from build123d import *

# Parameters (mm, degrees)
SKETCH1_W             = 425.069
SKETCH1_H             = 9.525
BOSS_EXTRUDE1_DEPTH   = 3.175
SKETCH2_W             = 3.175
SKETCH2_H             = 3.175
CUT_EXTRUDE1_DEPTH    = 213.611560649
SKETCH3_R             = 0.5
CUT_EXTRUDE2_DEPTH    = 213.611560649
SKETCH_PATTERN1_DEPTH = 3.175
SKETCH5_W             = 20
SKETCH5_H             = 3.18
BOSS_EXTRUDE2_DEPTH   = 3.175
SKETCH6_R             = 0.5
CUT_EXTRUDE3_DEPTH    = 213.706552841
SKETCH_PATTERN2_DEPTH = 3.175


# Read off the part's stored shape, not the designer's step: Sketch-Pattern1, Sketch-Pattern2
with BuildPart() as part:
    # Sketch1 → Boss-Extrude1 (new body)
    with BuildSketch(Plane(origin=(0, 0, 0), x_dir=(1, 0, 0), z_dir=(0, 1, 0))):
        Rectangle(SKETCH1_W, SKETCH1_H)
    extrude(amount=BOSS_EXTRUDE1_DEPTH)

    # Sketch2 → Cut-Extrude1 (cut, symmetric)
    with BuildSketch(Plane(origin=(0, 3.175, 0), x_dir=(1, 0, 0), z_dir=(0, 1, 0))):
        with Locations((-105.4735, 3.175)):
            Rectangle(SKETCH2_W, SKETCH2_H)
        with Locations((-210.947, 3.175)):
            Rectangle(SKETCH2_W, SKETCH2_H)
        with Locations((0, 3.175)):
            Rectangle(SKETCH2_W, SKETCH2_H)
    cut_extrude1 = extrude(amount=CUT_EXTRUDE1_DEPTH, both=True, mode=Mode.SUBTRACT)

    # Sketch3 → Cut-Extrude2 (cut, symmetric)
    with BuildSketch(Plane(origin=(0, 3.175, 0), x_dir=(1, 0, 0), z_dir=(0, 1, 0))):
        with Locations((-209.713053391, 1.941053391)):
            Circle(SKETCH3_R)
    cut_extrude2 = extrude(amount=CUT_EXTRUDE2_DEPTH, both=True, mode=Mode.SUBTRACT)

    # Mirror1: Cut-Extrude1 across plane
    add(cut_extrude1.mirror(Plane(origin=(0, 0, 0), x_dir=(0, 0, 1), z_dir=(1, 0, 0))), mode=Mode.SUBTRACT)

    # Sketch-Pattern1 outline → Sketch-Pattern1 (cut)
    with BuildSketch(Plane(origin=(0, 0, 0), x_dir=(1, 0, 0), z_dir=(0, 1, 0))):
        with BuildLine():
            Line((-103.886, 1.5875), (-104.593106781, 1.5875))
            ThreePointArc((-104.593106781, 1.5875), (-104.23955339, 1.441053391), (-103.886, 1.5875))
        make_face()
        with BuildLine():
            Line((-103.886, 2.294606781), (-103.886, 1.5875))
            ThreePointArc((-103.886, 1.5875), (-103.739553391, 1.941053391), (-103.886, 2.294606781))
        make_face()
        with BuildLine():
            Line((107.061, 1.5875), (106.353893219, 1.5875))
            ThreePointArc((106.353893219, 1.5875), (106.70744661, 1.441053391), (107.061, 1.5875))
        make_face()
        with BuildLine():
            Line((107.061, 2.294606781), (107.061, 1.5875))
            ThreePointArc((107.061, 1.5875), (107.207446609, 1.941053391), (107.061, 2.294606781))
        make_face()
        with BuildLine():
            Line((1.5875, 1.5875), (0.880393219, 1.5875))
            ThreePointArc((0.880393219, 1.5875), (1.23394661, 1.441053391), (1.5875, 1.5875))
        make_face()
        with BuildLine():
            Line((1.5875, 2.294606781), (1.5875, 1.5875))
            ThreePointArc((1.5875, 1.5875), (1.733946609, 1.941053391), (1.5875, 2.294606781))
        make_face()
    sketch_pattern1 = extrude(amount=SKETCH_PATTERN1_DEPTH, mode=Mode.SUBTRACT)

    # Mirror2: Cut-Extrude2, Sketch-Pattern1 across plane
    add(cut_extrude2.mirror(Plane(origin=(0, 0, 0), x_dir=(0, 0, 1), z_dir=(1, 0, 0))), mode=Mode.SUBTRACT)
    add(sketch_pattern1.mirror(Plane(origin=(0, 0, 0), x_dir=(0, 0, 1), z_dir=(1, 0, 0))), mode=Mode.SUBTRACT)

    # Sketch5 → Boss-Extrude2 (add)
    with BuildSketch(Plane(origin=(0, 3.175, 0), x_dir=(1, 0, 0), z_dir=(0, 1, 0))):
        with Locations((-158.21025, -6.3525)):
            Rectangle(SKETCH5_W, SKETCH5_H)
        with Locations((-52.73675, -6.3525)):
            Rectangle(SKETCH5_W, SKETCH5_H)
        with Locations((52.73675, -6.3525)):
            Rectangle(SKETCH5_W, SKETCH5_H)
        with Locations((158.21025, -6.3525)):
            Rectangle(SKETCH5_W, SKETCH5_H)
    extrude(amount=-BOSS_EXTRUDE2_DEPTH)

    # Sketch6 → Cut-Extrude3 (cut, symmetric)
    with BuildSketch(Plane(origin=(0, 3.175, 0), x_dir=(1, 0, 0), z_dir=(0, 1, 0))):
        with Locations((-168.563803391, -5.116053391)):
            Circle(SKETCH6_R)
    cut_extrude3 = extrude(amount=CUT_EXTRUDE3_DEPTH, both=True, mode=Mode.SUBTRACT)

    # Sketch-Pattern2 outline → Sketch-Pattern2 (cut)
    with BuildSketch(Plane(origin=(0, 0, 0), x_dir=(1, 0, 0), z_dir=(0, 1, 0))):
        with BuildLine():
            Line((-62.73675, -4.7625), (-62.73675, -5.469606781))
            ThreePointArc((-62.73675, -5.469606781), (-62.590303391, -5.116053391), (-62.73675, -4.7625))
        make_face()
        with BuildLine():
            Line((-63.443856781, -4.7625), (-62.73675, -4.7625))
            ThreePointArc((-62.73675, -4.7625), (-63.09030339, -4.616053391), (-63.443856781, -4.7625))
        make_face()
        with BuildLine():
            Line((148.21025, -4.7625), (148.21025, -5.469606781))
            ThreePointArc((148.21025, -5.469606781), (148.356696609, -5.116053391), (148.21025, -4.7625))
        make_face()
        with BuildLine():
            Line((147.503143219, -4.7625), (148.21025, -4.7625))
            ThreePointArc((148.21025, -4.7625), (147.85669661, -4.616053391), (147.503143219, -4.7625))
        make_face()
        with BuildLine():
            Line((42.73675, -4.7625), (42.73675, -5.469606781))
            ThreePointArc((42.73675, -5.469606781), (42.883196609, -5.116053391), (42.73675, -4.7625))
        make_face()
        with BuildLine():
            Line((42.029643219, -4.7625), (42.73675, -4.7625))
            ThreePointArc((42.73675, -4.7625), (42.38319661, -4.616053391), (42.029643219, -4.7625))
        make_face()
    sketch_pattern2 = extrude(amount=SKETCH_PATTERN2_DEPTH, mode=Mode.SUBTRACT)

    # Mirror3: Cut-Extrude3, Sketch-Pattern2 across plane
    add(cut_extrude3.mirror(Plane(origin=(0, 0, 0), x_dir=(0, 0, 1), z_dir=(1, 0, 0))), mode=Mode.SUBTRACT)
    add(sketch_pattern2.mirror(Plane(origin=(0, 0, 0), x_dir=(0, 0, 1), z_dir=(1, 0, 0))), mode=Mode.SUBTRACT)


solid = part.part
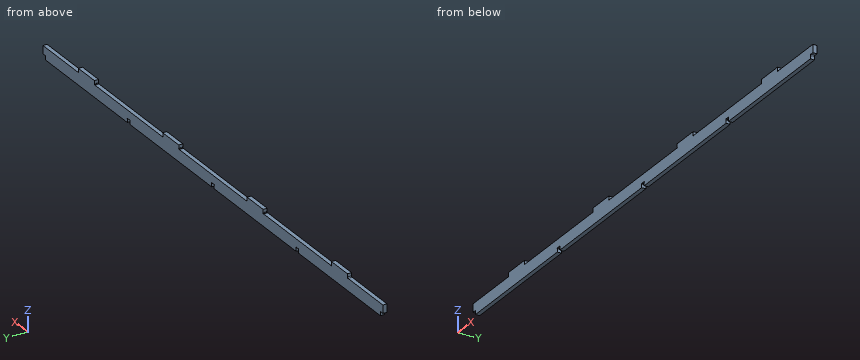
The listing builds one solid part. Answer for the finished solid, in the listing's coordinates (mm). Coordinates: 2 decimals unless noted, no trailing zeros. Loops run counter-clockwise (first coordinate to the right, second up) from the corner with the lowest first, then second, coordinate; pieces in that order, holes last.
1) Find the intervals of material crossed by L1, parallel to X at y = 2.5, z = -2; L2, parallel to X at y = 2.1, z = -3; L3, parallel to Z at x = 116, y = 1.5, in increasing order.
2) Flat-ended cylindrical pins translate along their axes: pin 1 Ø0.9 at (x, y) = (105, 1) entering from -Z; pin 2 Ø1.2 at (y, z) = (2, -3) entering from +X; pin 3 Ø1.2 at (y, z) = (2, -3) entering from -X. Find the tip coordinate at first contact, or state that the pin passes through.
3) Find section A-A on x = 113. Write down the section's boundary in (y, z) (1 decimal), then the cut area to 3 significant figures.
Values:
1. L1: x = -209.22 to -107.2, -103.74 to -1.73, 1.73 to 103.74, 107.2 to 209.22
1. L2: x = -209.36 to -107.06, -103.89 to -1.59, 1.59 to 103.89, 107.06 to 209.36
1. L3: z = -4.76 to 4.76
2. pin 1: stops at z = -1.59
2. pin 2: stops at x = 209.36
2. pin 3: stops at x = -209.36
3. outline: (0, -4.8) - (3.2, -4.8) - (3.2, 4.8) - (0, 4.8) - close
3. area: 30.2 mm2
